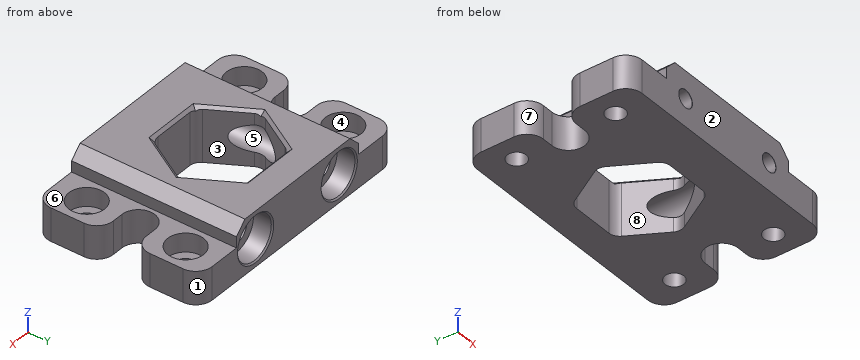
from build123d import *

# Parameters (mm, degrees)
SKETCH1_W                                           = 46
SKETCH1_H                                           = 30
BOSS_EXTRUDE1_DEPTH                                 = 10
CUT_EXTRUDE1_DEPTH                                  = 56.821142948
CBORE_FOR_M5_HEX_SOCKET_HEAD_CAP_SCR_2_COUNT        = 2
CBORE_FOR_M5_HEX_SOCKET_HEAD_CAP_SCR_2_PITCH        = 19.629909152
CBORE_FOR_M3_HEX_SOCKET_HEAD_CAP_SCR_2_COUNT        = 2
CBORE_FOR_M3_HEX_SOCKET_HEAD_CAP_SCR_2_PITCH        = 37
CBORE_FOR_M3_HEX_SOCKET_HEAD_CAP_SCR_3_COUNT        = 2
CBORE_FOR_M3_HEX_SOCKET_HEAD_CAP_SCR_3_PITCH        = 41.146081223
CBORE_FOR_M3_HEX_SOCKET_HEAD_CAP_SCR_4_COUNT        = 2
CBORE_FOR_M3_HEX_SOCKET_HEAD_CAP_SCR_4_PITCH        = 18
TAP_DRILL_FOR_M3_HELICOIL1_D                        = 3.15
TAP_DRILL_FOR_M3_HELICOIL1_DEPTH                    = 24.053644525
TAP_DRILL_FOR_M3_HELICOIL1_CSINK_D                  = 3.2
TAP_DRILL_FOR_M3_HELICOIL1_CSINK_ANGLE              = 90
TAP_DRILL_FOR_M3_HELICOIL1_TIP                      = 0.946355475
CUT_EXTRUDE2_DEPTH                                  = 56.821142948
CUT_EXTRUDE3_DEPTH                                  = 4
CBORE_FOR_M3_HEX_SOCKET_HEAD_CAP_SCREW2_D           = 3.4
CBORE_FOR_M3_HEX_SOCKET_HEAD_CAP_SCREW2_CBORE_D     = 6.5
CBORE_FOR_M3_HEX_SOCKET_HEAD_CAP_SCREW2_CBORE_DEPTH = 3.4
CHAMFER1_SIZE                                       = 2
CHAMFER2_SIZE                                       = 0.5
FILLET2_R                                           = 2
FILLET1_R                                           = 3


with BuildPart() as part:
    # Sketch1 → Boss-Extrude1 (new body)
    with BuildSketch(Plane.XY):
        with Locations((23, 15)):
            Rectangle(SKETCH1_W, SKETCH1_H)
    extrude(amount=BOSS_EXTRUDE1_DEPTH)

    # Sketch2 → Cut-Extrude1 (cut, through all)
    with BuildSketch(Plane.XY.offset(10)):
        Polygon((27.907477288, 24.5), (18.092522712, 24.5), (13.185045424, 16), (18.092522712, 7.5), (27.907477288, 7.5), (32.814954576, 16), align=None)
    extrude(amount=-CUT_EXTRUDE1_DEPTH, mode=Mode.SUBTRACT)

    # Sketch4 → CBORE for M5 Hex Socket Head Cap Screw1 (revolve, cut)
    with BuildSketch(Plane(origin=(13.185045424, 30, 5), x_dir=(0, 0, 1), z_dir=(1, 0, 0))):
        Polygon((0, 0), (0, 27), (2.5, 25.497848452), (2.5, 3.5), (4, 3.5), (4, 0.25), (4.25, 0), align=None)
    cbore_for_m5_hex_socket_head_cap_screw1 = revolve(axis=Axis((13.185045424, 36.35, 5), (0, -1, 0)), mode=Mode.SUBTRACT)

    # CBORE for M5 Hex Socket Head Cap Scr 2: CBORE for M5 Hex Socket Head Cap Screw1 ×2
    with Locations(*[(i * CBORE_FOR_M5_HEX_SOCKET_HEAD_CAP_SCR_2_PITCH, 0, 0) for i in range(1, CBORE_FOR_M5_HEX_SOCKET_HEAD_CAP_SCR_2_COUNT)]):
        add(cbore_for_m5_hex_socket_head_cap_screw1, mode=Mode.SUBTRACT)

    # Sketch6 → CBORE for M3 Hex Socket Head Cap Screw1 (revolve, cut)
    with BuildSketch(Plane(origin=(4.5, 24, 10), x_dir=(0, -1, 0), z_dir=(1, 0, 0))):
        Polygon((0, 0), (0, 10), (1.7, 10), (1.7, 3.4), (3.25, 3.4), (3.25, 0.025), (3.275, 0), align=None)
    cbore_for_m3_hex_socket_head_cap_screw1 = revolve(axis=Axis((4.5, 24, 16.35), (0, 0, -1)), mode=Mode.SUBTRACT)

    # CBORE for M3 Hex Socket Head Cap Scr 2: CBORE for M3 Hex Socket Head Cap Screw1 ×2
    with Locations(*[(i * CBORE_FOR_M3_HEX_SOCKET_HEAD_CAP_SCR_2_PITCH, 0, 0) for i in range(1, CBORE_FOR_M3_HEX_SOCKET_HEAD_CAP_SCR_2_COUNT)]):
        add(cbore_for_m3_hex_socket_head_cap_screw1, mode=Mode.SUBTRACT)

    # CBORE for M3 Hex Socket Head Cap Scr 3: CBORE for M3 Hex Socket Head Cap Screw1 ×2
    with Locations(*[Vector(0.8992350887457975, -0.4374657188493034, 0) * (i * CBORE_FOR_M3_HEX_SOCKET_HEAD_CAP_SCR_3_PITCH) for i in range(1, CBORE_FOR_M3_HEX_SOCKET_HEAD_CAP_SCR_3_COUNT)]):
        add(cbore_for_m3_hex_socket_head_cap_screw1, mode=Mode.SUBTRACT)

    # CBORE for M3 Hex Socket Head Cap Scr 4: CBORE for M3 Hex Socket Head Cap Screw1 ×2
    with Locations(*[(0, -i * CBORE_FOR_M3_HEX_SOCKET_HEAD_CAP_SCR_4_PITCH, 0) for i in range(1, CBORE_FOR_M3_HEX_SOCKET_HEAD_CAP_SCR_4_COUNT)]):
        add(cbore_for_m3_hex_socket_head_cap_screw1, mode=Mode.SUBTRACT)

    # Tap Drill for M3 Helicoil1
    with Locations(Plane(origin=(0, 0, 0), x_dir=(-1, 0, 0), z_dir=(0, -1, 0))):
        with Locations((-13.185045424, -5), (-32.814954576, -5)):
            CounterSinkHole(TAP_DRILL_FOR_M3_HELICOIL1_D / 2, TAP_DRILL_FOR_M3_HELICOIL1_CSINK_D / 2, depth=TAP_DRILL_FOR_M3_HELICOIL1_DEPTH, counter_sink_angle=TAP_DRILL_FOR_M3_HELICOIL1_CSINK_ANGLE)
            with Locations((0, 0, -(TAP_DRILL_FOR_M3_HELICOIL1_DEPTH + TAP_DRILL_FOR_M3_HELICOIL1_TIP / 2))):  # 118° drill point
                Cone(0, TAP_DRILL_FOR_M3_HELICOIL1_D / 2, TAP_DRILL_FOR_M3_HELICOIL1_TIP, mode=Mode.SUBTRACT)

    # Sketch11 → Cut-Extrude2 (cut, through all)
    with BuildSketch(Plane.XY.offset(10)):
        with BuildLine():
            ThreePointArc((5, 12), (8, 15), (5, 18))
            Line((5, 18), (0, 18))
            Line((0, 18), (0, 12))
            Line((0, 12), (5, 12))
        make_face()
        with BuildLine():
            Line((46, 12), (46, 18))
            Line((46, 18), (41, 18))
            ThreePointArc((41, 18), (38, 15), (41, 12))
            Line((41, 12), (46, 12))
        make_face()
    extrude(amount=-CUT_EXTRUDE2_DEPTH, mode=Mode.SUBTRACT)

    # Sketch13 → Cut-Extrude3 (cut)
    with BuildSketch(Plane.XY.offset(10)):
        with BuildLine():
            Line((8.685045424, 0), (8.685045424, 30))
            Line((8.685045424, 30), (0, 30))
            Line((0, 30), (0, 18))
            Line((0, 18), (5, 18))
            ThreePointArc((5, 18), (8, 15), (5, 12))
            Line((5, 12), (0, 12))
            Line((0, 12), (0, 0))
            Line((0, 0), (8.685045424, 0))
        make_face()
        with BuildLine():
            Line((46, 30), (37.314954576, 30))
            Line((37.314954576, 30), (37.314954576, 0))
            Line((37.314954576, 0), (46, 0))
            Line((46, 0), (46, 12))
            Line((46, 12), (41, 12))
            ThreePointArc((41, 12), (38, 15), (41, 18))
            Line((41, 18), (46, 18))
            Line((46, 18), (46, 30))
        make_face()
    extrude(amount=-CUT_EXTRUDE3_DEPTH, mode=Mode.SUBTRACT)

    # CBORE for M3 Hex Socket Head Cap Screw2 (through all)
    with Locations(Plane.XY.offset(6)):
        with Locations((4.5, 24), (4.5, 6), (41.5, 24), (41.5, 6)):
            CounterBoreHole(CBORE_FOR_M3_HEX_SOCKET_HEAD_CAP_SCREW2_D / 2, CBORE_FOR_M3_HEX_SOCKET_HEAD_CAP_SCREW2_CBORE_D / 2, CBORE_FOR_M3_HEX_SOCKET_HEAD_CAP_SCREW2_CBORE_DEPTH)

    # Chamfer1
    chamfer1_edges = [part.edges().sort_by_distance(p)[0] for p in [
        (8.685045424, 15, 10),
        (37.314954576, 15, 10),
    ]]
    chamfer(chamfer1_edges, length=CHAMFER1_SIZE)

    # Chamfer2
    chamfer2_edges = [part.edges().sort_by_distance(p)[0] for p in [
        (30.361215932, 20.25, 10),
        (23, 24.5, 10),
        (15.638784068, 20.25, 10),
        (15.638784068, 11.75, 10),
        (23, 7.5, 10),
        (30.361215932, 11.75, 10),
    ]]
    chamfer(chamfer2_edges, length=CHAMFER2_SIZE)

    # Fillet2
    fillet2_edges = [part.edges().sort_by_distance(p)[0] for p in [
        (32.814954576, 16, 8.5),
        (32.814954576, 16, 1.25),
        (27.907477288, 7.5, 4.75),
        (18.092522712, 7.5, 4.75),
        (13.185045424, 16, 1.25),
        (13.185045424, 16, 8.5),
        (18.092522712, 24.5, 4.75),
        (27.907477288, 24.5, 4.75),
    ]]
    fillet(fillet2_edges, radius=FILLET2_R)

    # Fillet1
    fillet1_edges = [part.edges().sort_by_distance(p)[0] for p in [
        (0, 12, 3),
        (0, 18, 3),
        (46, 18, 3),
        (46, 12, 3),
        (0, 30, 3),
        (46, 30, 3),
        (46, 0, 3),
        (0, 0, 3),
    ]]
    fillet(fillet1_edges, radius=FILLET1_R)


solid = part.part
Geometry check sheet. Reference: the model listing, model coordinates, mm. Face numbers are marked on the shaded views. A direction names the side the tool comes from. Give positions to 0.01 mm unless a question says otherwise; leave off trailing zeros. Order: outer loops, then holes, each group sorted by start corner. A loop starts at its lowest first (then second) coordinate and runs counter-clockwise, first axis right, second up.
1) Cross-section at B-B (y = 6). Record the boundary of the cut face in (x, z), then the cut area to 3 significant figures.
Results are:
outline: (0, 0) - (2.8, 0) - (2.8, 2.6) - (1.25, 2.6) - (1.25, 6) - (0, 6) - close; (6.2, 0) - (39.8, 0) - (39.8, 2.6) - (38.25, 2.6) - (38.25, 6) - (37.31, 6) - (37.31, 8) - (35.31, 10) - (10.69, 10) - (8.69, 8) - (8.69, 6) - (7.75, 6) - (7.75, 2.6) - (6.2, 2.6) - close; (43.2, 0) - (46, 0) - (46, 6) - (44.75, 6) - (44.75, 2.6) - (43.2, 2.6) - close; hole circle Ø5 at (13.19, 5); hole circle Ø5 at (32.81, 5)
area: 285 mm2
2) Material ranges on probe 1 along Y at (x, z) = (41.5, 4.2); probe 2 along X at (y, z) = (6, 1.45); probe 3 along Y at (x, z) = (26, 8.25), recorded low to high.
Results are:
probe 1: y = 0 to 2.75, 9.25 to 12, 18 to 20.75, 27.25 to 30
probe 2: x = 0 to 2.8, 6.2 to 39.8, 43.2 to 46
probe 3: y = 0 to 7.5, 24.5 to 30
3) Cross-section at A-A (x = 4.5). Record the boundary of the cut face in (y, z), then the cut area to 3 significant figures.
Results are:
outline: (0, 0) - (4.3, 0) - (4.3, 2.6) - (2.75, 2.6) - (2.75, 6) - (0, 6) - close; (7.7, 0) - (12, 0) - (12, 6) - (9.25, 6) - (9.25, 2.6) - (7.7, 2.6) - close; (18, 0) - (22.3, 0) - (22.3, 2.6) - (20.75, 2.6) - (20.75, 6) - (18, 6) - close; (25.7, 0) - (30, 0) - (30, 6) - (27.25, 6) - (27.25, 2.6) - (25.7, 2.6) - close
area: 82.1 mm2
4) Tool access check on the marked faces 4, 5, 6, 7 and 8. Record the directions out of +Z, -Z, +X, -X, +Y, -Y that give a thin tool (end or side, any length) a straight path to the whole face; none if there is none.
Results are:
face 4: +Z
face 5: +Y
face 6: +Z, +X, +Y, -Y
face 7: +Z, -Z, -X
face 8: +Z, -Z
5) Cross-section at C-C (z = 2). Give the number of separate pieces and of enclosed holes in the cut face, then the cut area to 3 significant figures.
Results are:
separate pieces: 1
enclosed holes: 5
area: 954 mm2
6) Gauge pin test, flat ends, axial feed: pin 1 (4.5 mm diameter, centred on x = 4.5, y = 20, fed in from +Z); pin 2 (4 mm diameter, centred on x = 32.81, z = 5, fed in from +Y); pin 3 (2 mm diameter, centred on x = 41.5, y = 24, fed in from +Z); pin 4 (1 mm diameter, centred on y = 4.5, z = 7, fed in from -X). Record the tip position at first contact, or that the pin passes through.
Results are:
pin 1: stops at z = 6
pin 2: stops at y = 4.2
pin 3: passes through
pin 4: stops at x = 8.69
7) Draft check along Y on the marked faces 1, 2 and 3. Enter one of: released by +Y, released by -Y, zero draft, split by the parting line, or undercut.
Results are:
face 1: released by +Y
face 2: released by -Y
face 3: undercut
